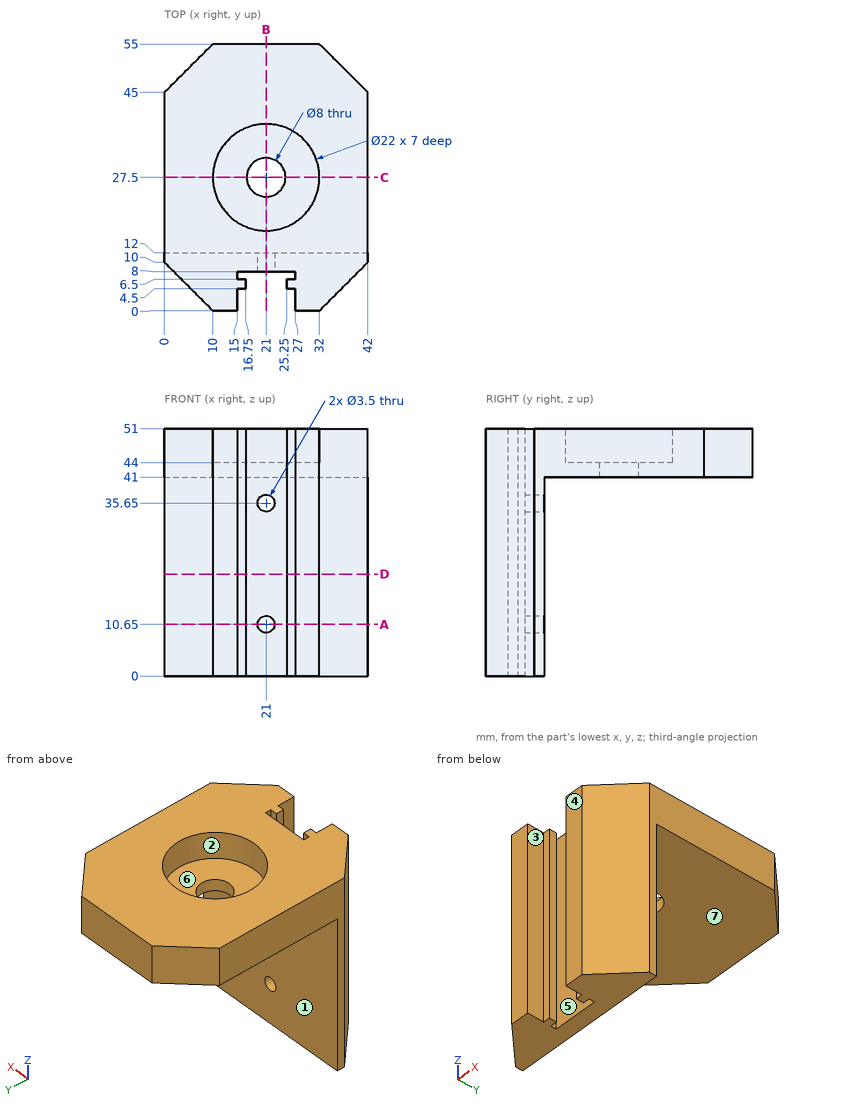
Design review of the part shown in the three views and the two pictorial views. Dimensions are in mm from the part's minimum x, y and z. A direction names the side the tool comes from. Round coordinates to 2 decimals unless told otherwise and drop trailing zeros. Loops run counter-clockwise (first coordinate to the right, second up) from the corner with the lowest first, then second, coordinate; pieces in that order, holes last. Notation, with made-up numbers: (-35.5, -30.5) - (-9.5, -30.5) arc R13 cw to (-9.5, -11.5) - close; hole circle Ø5 at (-21, -6). An arc over 180 degrees is marked (long way). Write each question's results on one line, items separated by ' | '. Start each with the question number.
Q1. Draft analysis for pull direction Y (two halves, no side actions). For the marked faces 1, 2, 3 and 4, state which applies: pulls with the +Y half, pulls with the -Y half, needs draft (parallel to the pull), parting line crosses it, or undercut.
Q2. Take a section at A-A on z = 10.65. Give the boundary of the cut face in (x, y), plus the area to 3 significant figures.
Q3. Take a section at B-B on x = 21. Give the boundary of the cut face in (y, z).
Q4. Wall thickness on line 1 along Z through (x, y) = (21, 10); line 2 along Y through (x, z) = (26.5, 12); line 3 along Y through (x, z) = (21, 43.1): over which ranges is each line inside the solid? List them lowest first. Write a range as [from, to].
Q5. Take a section at C-C on y = 27.5. Give the boundary of the cut face in (x, z), plus the area to 3 significant figures.
Q6. Insertion check: P1, Ø4, axis at x = 15, y = 46.5, coming from the -Z side; P2, Ø0.9, axis at x = 16, z = 14.5, coming from the -Y side; P3, Ø1.9, axis at x = 15.5, z = 24, coming from the +Y side. Each pin has a flat end and moves straight along its axis. Give the tip position at first contact, or say it passes through.
Q7. Tool access review of the marked faces 5, 6 and 7: name each direction out of +Z, -Z, +X, -X, +Y, -Y from which nothing blocks a thin tool from reaching the whole face with its end or side.
Q8. Take a section at D-D on z = 21. Give the boundary of the cut face in (x, y), plus the area to 3 significant figures.
Data:
1) face 1: pulls with the +Y half | face 2: undercut | face 3: needs draft | face 4: pulls with the -Y half
2) outline: (0, 10) - (10, 0) - (15, 0) - (15, 4.5) - (16.75, 4.5) - (16.75, 6.5) - (15, 6.5) - (15, 8) - (19.25, 8) - (19.25, 12) - (0, 12) - close; (22.75, 8) - (27, 8) - (27, 6.5) - (25.25, 6.5) - (25.25, 4.5) - (27, 4.5) - (27, 0) - (32, 0) - (42, 10) - (42, 12) - (22.75, 12) - close | area: 301 mm²
3) outline: (8, 0) - (12, 0) - (12, 8.9) - (8, 8.9) - close; (8, 12.4) - (12, 12.4) - (12, 33.9) - (8, 33.9) - close; (8, 37.4) - (12, 37.4) - (12, 41) - (23.5, 41) - (23.5, 44) - (16.5, 44) - (16.5, 51) - (8, 51) - close; (31.5, 41) - (55, 41) - (55, 51) - (38.5, 51) - (38.5, 44) - (31.5, 44) - close
4) line 1: z = [0, 8.9], [12.4, 33.9], [37.4, 51] | line 2: y = [4.5, 6.5], [8, 12] | line 3: y = [8, 23.5], [31.5, 55]
5) outline: (0, 41) - (17, 41) - (17, 44) - (10, 44) - (10, 51) - (0, 51) - close; (25, 41) - (42, 41) - (42, 51) - (32, 51) - (32, 44) - (25, 44) - close | area: 242 mm²
6) P1: stops at z = 41 | P2: stops at y = 4.5 | P3: stops at y = 12
7) face 5: +Z, -Z | face 6: +Z | face 7: -Z, +X, -X, +Y
8) outline: (0, 10) - (10, 0) - (15, 0) - (15, 4.5) - (16.75, 4.5) - (16.75, 6.5) - (15, 6.5) - (15, 8) - (27, 8) - (27, 6.5) - (25.25, 6.5) - (25.25, 4.5) - (27, 4.5) - (27, 0) - (32, 0) - (42, 10) - (42, 12) - (0, 12) - close | area: 315 mm²
